```python
from build123d import *

# Parameters (mm, degrees)
SKETCH_W        = 40
SKETCH_H        = 35
PAD_DEPTH       = 6
SKETCH002_W     = 40
SKETCH002_H     = 17
PAD001_DEPTH    = 3
SKETCH001_R     = 1.9
SKETCH001_R_2   = 1.6
POCKET_DEPTH    = 9.001
SKETCH003_W     = 14
SKETCH003_H     = 35
PAD002_DEPTH    = 13
SKETCH004_W     = 11
SKETCH004_H     = 23.4
POCKET001_DEPTH = 19
SKETCH005_R     = 0.75
POCKET002_DEPTH = 10
SKETCH006_W     = 2
SKETCH006_H     = 6
POCKET003_DEPTH = 8
SKETCH007_W     = 5
SKETCH007_H     = 18
POCKET004_DEPTH = 2.5


with BuildPart() as part:
    # Sketch → Pad (new body)
    with BuildSketch(Plane.XY):
        with Locations((0, -0.5)):
            Rectangle(SKETCH_W, SKETCH_H)
    extrude(amount=PAD_DEPTH)

    # Sketch002 (on Face5 of Pad) → Pad001 (join)
    with BuildSketch(Plane(origin=(0, 0, 0), x_dir=(1, 0, 0), z_dir=(0, 0, -1))):
        with Locations((0, -8.5)):
            Rectangle(SKETCH002_W, SKETCH002_H)
    extrude(amount=PAD001_DEPTH)

    # Sketch001 (on Face6 of Pad) → Pocket (cut, through all)
    with BuildSketch(Plane.XY.offset(6)):
        with Locations((-15, 5)):
            Circle(SKETCH001_R)
        with Locations((15, 5)):
            Circle(SKETCH001_R)
        with Locations((0, -5)):
            Circle(SKETCH001_R_2)
    extrude(amount=-POCKET_DEPTH, mode=Mode.SUBTRACT)

    # Sketch003 (on Face1 of Pocket) → Pad002 (join)
    with BuildSketch(Plane.XY.offset(6)):
        with Locations((13, -0.5)):
            Rectangle(SKETCH003_W, SKETCH003_H)
    extrude(amount=PAD002_DEPTH)

    # Sketch004 (on Face9 of Pad002) → Pocket001 (cut)
    with BuildSketch(Plane.XY.offset(19)):
        with Locations((14.5, -0.5)):
            Rectangle(SKETCH004_W, SKETCH004_H)
    extrude(amount=-POCKET001_DEPTH, mode=Mode.SUBTRACT)

    # Sketch005 (on Face12 of Pocket001) → Pocket002 (cut)
    with BuildSketch(Plane.XY.offset(19)):
        with Locations((15, 13.5)):
            Circle(SKETCH005_R)
        with Locations((15, -14.5)):
            Circle(SKETCH005_R)
    extrude(amount=-POCKET002_DEPTH, mode=Mode.SUBTRACT)

    # Sketch006 (on Face11 of Pocket002) → Pocket003 (cut)
    with BuildSketch(Plane.YZ.offset(20)):
        with Locations((12.2, 3)):
            Rectangle(SKETCH006_W, SKETCH006_H)
    extrude(amount=-POCKET003_DEPTH, mode=Mode.SUBTRACT)

    # Sketch007 (on Face10 of Pocket003) → Pocket004 (cut)
    with BuildSketch(Plane(origin=(0, 0, 0), x_dir=(1, 0, 0), z_dir=(0, 0, -1))):
        with Locations((0, 9)):
            Rectangle(SKETCH007_W, SKETCH007_H)
    extrude(amount=-POCKET004_DEPTH, mode=Mode.SUBTRACT)


solid = part.part
```
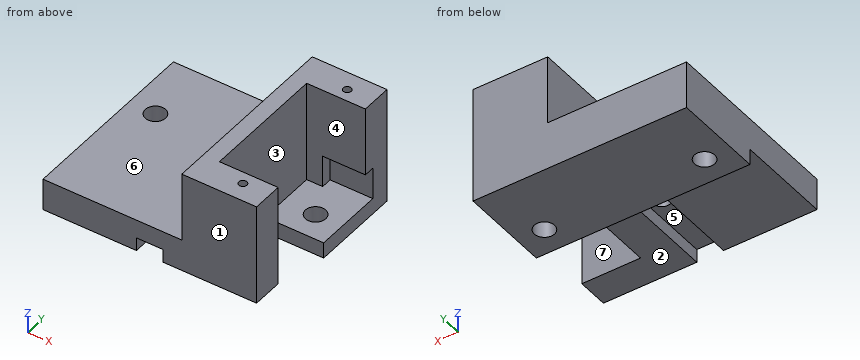
Can you work these out from the model? Positions are in its coordinate system, mm. Face numbers are marked on the shaded views. A direction names the side the tool comes from. Coordinates: 2 decimals unless noted, no trailing zeros. Order: outer loops, then holes, each group sorted by start corner. A loop starts at its lowest first (then second) coordinate and runs counter-clockwise, first axis right, second up. Notation, with made-up numbers: (35, 2.25) - (75, 2.25) arc R15 cw to (75, 28.25) - close; hole circle Ø10 at (7, 22). An arc over 180 degrees is marked (long way). Answer in a Markdown table with one row per item.
1. Suppose I cut it at B-B (y = 5). Please give me the cut outline in (x, z).
Reply:
| item | result |
|---|---|
| outline | (-20, -3) - (-16.9, -3) - (-16.9, 6) - (-20, 6) - close; (-13.1, -3) - (13.1, -3) - (13.1, 0) - (9, 0) - (9, 19) - (6, 19) - (6, 6) - (-13.1, 6) - close; (16.9, -3) - (20, -3) - (20, 0) - (16.9, 0) - close |
2. For pin 1 (14 mm diameter, centred on x = 9.5, y = -6.5, fed in from -Z); pin 2 (1.6 mm diameter, centred on y = 12, z = 4, fed in from +X); pin 3 (6.5 mm diameter, centred on y = 0, z = 13, fed in from -X); pin 4 (3 mm diameter, centred on x = -15, y = 5, fed in from -Z), each with a flat end and sliding along its axis, tell me the tip position at first contact or that it passes through.
Reply:
| item | result |
|---|---|
| pin 1 | stops at z = -3 |
| pin 2 | stops at x = 12 |
| pin 3 | stops at x = 6 |
| pin 4 | passes through |
3. For the marked faces 4, 5, 6 and 7, which set-ups out of +Z, -Z, +X, -X, +Y, -Y let a thin tool reach every point of the face, with its end or its side?
Reply:
| item | result |
|---|---|
| face 4 | +Z, +X |
| face 5 | -Z, -Y |
| face 6 | +Z, -X, +Y, -Y |
| face 7 | +Z, -Z, +X |
4. If I drill on line 1 along Y through (x, z) = (15, 14.25); line 2 along Y through (x, z) = (15, -1.4); line 3 along Y through (x, z) = (-15, 2.25), over which ranges is the centre line in solid material (lowest first)?
Reply:
| item | result |
|---|---|
| line 1 | y = -18 to -15.25, -13.75 to -12.2, 11.2 to 12.75, 14.25 to 17 |
| line 2 | y = 0 to 3.1, 6.9 to 17 |
| line 3 | y = -18 to 3.1, 6.9 to 17 |
5. Suppose I cut it at A-A (x = 0). Please give me the cut outline in (y, z).
Reply:
| item | result |
|---|---|
| outline | (-18, 2.5) - (-6.6, 2.5) - (-6.6, 6) - (-18, 6) - close; (-3.4, 2.5) - (0, 2.5) - (0, -3) - (17, -3) - (17, 6) - (-3.4, 6) - close |
6. If we mould it in two halves opening along Y, with no side actions, what happens to the marked faces 1, 2 and 3? For each: pulls with the +Y half, pulls with the -Y half, needs draft (parallel to the pull), parting line crosses it, or undercut.
Reply:
| item | result |
|---|---|
| face 1 | pulls with the -Y half |
| face 2 | needs draft |
| face 3 | undercut |
7. Suppose I cut it at C-C (x = 15). Please give me the cut outline in (y, z), and give its area (3 significant figures).
Reply:
| item | result |
|---|---|
| outline | (-18, 0) - (-12.2, 0) - (-12.2, 19) - (-13.75, 19) - (-13.75, 9) - (-15.25, 9) - (-15.25, 19) - (-18, 19) - close; (0, -3) - (3.1, -3) - (3.1, 0) - (0, 0) - close; (6.9, -3) - (17, -3) - (17, 19) - (14.25, 19) - (14.25, 9) - (12.75, 9) - (12.75, 19) - (11.2, 19) - (11.2, 6) - (13.2, 6) - (13.2, 0) - (6.9, 0) - close |
| area | 218 mm^2 |
8. Suppose I cut it at D-D (z = -1.5). Please give me the cut outline in (x, y), and give its area (3 significant figures).
Reply:
| item | result |
|---|---|
| outline | (-20, 0) - (20, 0) - (20, 17) - (-20, 17) - close; hole circle Ø3.8 at (-15, 5); hole circle Ø3.8 at (15, 5) |
| area | 657 mm^2 |
